Check sheet for the modelled part. Datum: model origin and axes. Units: mm. Give positions to 0.01 mm unless a question says otherwise; leave off trailing zeros. Write each loop counter-clockwise with the first axis right and the second up, starting at its lowest first coordinate (ties: lowest second). Pieces come first, ordered by that corner, then holes. Notation, with made-up numbers: (33, -8.5) -> (42, -8.5) arc R29 ccw to (42, 13.5) -> close; hole circle Ø3 at (27.25, -9.5). An arc over 180 degrees is marked (long way). Return JSON: item names as keys, results as strings.
from build123d import *

# Parameters (mm, degrees)
F1_DEPTH = 4


with BuildPart() as f1:
    # F0 (on Top) → F1 (new body)
    with BuildSketch(Plane.XY):
        with BuildLine():
            Line((-9.5, 57.454867), (-9.5, 37.454867))
            ThreePointArc((-9.5, 37.454867), (-8.110527, 29.236411), (-4.096559, 21.931501))
            ThreePointArc((-4.096559, 21.931501), (-3.276878, 19.270544), (-3, 16.5))
            Line((-3, 16.5), (-3, 0))
            Line((-3, 0), (0, 0))
            Line((0, 0), (0, 57.454867))
            Line((0, 57.454867), (-9.5, 57.454867))
        make_face()
    extrude(amount=F1_DEPTH)

    # F2: F1 across face


with BuildPart() as f1_1:
    add(f1.part)
    add(f1.part.mirror(Plane(origin=(-1.5, 0, 2), x_dir=(1, 0, 0), z_dir=(0, -1, 0))))

    # F3: F1 across face


with BuildPart() as f1_2:
    add(f1_1.part)
    add(f1_1.part.mirror(Plane(origin=(0, 0, 2), x_dir=(0, 1, 0), z_dir=(1, 0, 0))))


solid = f1_2.part
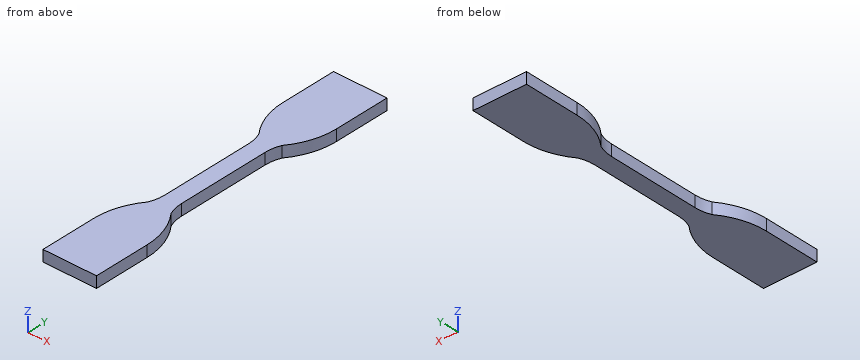
(1) Thickness scan on L1, parallel to X at y = 12, z = 0.3; L2, parallel to Y at x = -7, z = 2.7; L3, parallel to Y at x = -5, z = 0.7. Record the ranges inside material, lowest first.
Reply:
{"L1": "-3 to 3", "L2": "-57.45 to -26.56, 26.56 to 57.45", "L3": "-57.45 to -23.15, 23.15 to 57.45"}
(2) Cross-section at B-B on z = 1.35. Enter the section's corners in (x, y).
Reply:
{"outline": "(-9.5, -57.45) -> (9.5, -57.45) -> (9.5, -37.45) arc R25 ccw to (4.1, -21.93) arc R14 cw to (3, -16.5) -> (3, 16.5) arc R14 cw to (4.1, 21.93) arc R25 ccw to (9.5, 37.45) -> (9.5, 57.45) -> (-9.5, 57.45) -> (-9.5, 37.45) arc R25 ccw to (-4.1, 21.93) arc R14 cw to (-3, 16.5) -> (-3, -16.5) arc R14 cw to (-4.1, -21.93) arc R25 ccw to (-9.5, -37.45) -> close"}
(3) Depth check by flat-ended pin: pin 1 Ø2 at (x, y) = (5, -25.5) entering from -Z; pin 2 Ø2 at (y, z) = (5.5, 2.5) entering from +X; pin 3 Ø2 at (y, z) = (-4, 3) entering from -X. Enter the tip coordinate at first touch or a pass-through.
Reply:
{"pin 1": "z = 0", "pin 2": "x = 3", "pin 3": "x = -3"}
(4) Cross-section at D-D on y = -14.5. Enter the section's corners in (x, z).
Reply:
{"outline": "(-3, 0) -> (3, 0) -> (3, 4) -> (-3, 4) -> close"}
(5) Cross-section at C-C on x = -6. Enter the section's corners in (y, z), then the cut area to 3 significant figures.
Reply:
{"outline": "(-57.45, 0) -> (-24.7, 0) -> (-24.7, 4) -> (-57.45, 4) -> close; (24.7, 0) -> (57.45, 0) -> (57.45, 4) -> (24.7, 4) -> close", "area": "262 mm^2"}
(6) Cross-section at A-A on x = 6.5. Enter the section's corners in (y, z), then the cut area to 3 significant figures.
Reply:
{"outline": "(-57.45, 0) -> (-25.58, 0) -> (-25.58, 4) -> (-57.45, 4) -> close; (25.58, 0) -> (57.45, 0) -> (57.45, 4) -> (25.58, 4) -> close", "area": "255 mm^2"}
